Autodesk Inventor part; units mm, degrees
ref_plane "YZ Plane" through (0, 0, 0) normal (1, 0, 0) x (0, 1, 0)
ref_plane "XZ Plane" through (0, 0, 0) normal (0, 1, 0) x (-1, 0, 0)
ref_plane "XY Plane" through (0, 0, 0) normal (0, 0, 1) x (1, 0, 0)
sketch "Sketch1" plane through (0, 0, 0) normal (0, 1, 0) x (-1, 0, 0)
  line L0 (42.5, -32.5) -> (-42.5, -32.5)
  line L1 (-42.5, -32.5) -> (-42.5, 32.5)
  line L2 (-42.5, 32.5) -> (42.5, 32.5)
  line L3 (42.5, 32.5) -> (42.5, -32.5)
  point P0 (0, 0)
  point P1 (42.5, 0)
  point P2 (0, -32.5)
  dimension "d0" = 85
  dimension "d1" = 65
extrude "Extrusion1" add sketch "Sketch1" along normal blind 40
sketch "Sketch2" plane through (0, 40, 0) normal (0, 1, 0) x (1, 0, 0)
  point P0 (0, 0)
shell "Shell1" thickness 1 removed faces 1 at (14.1667, 40, 10.8333)
sketch "Sketch4" plane through (-42.5, 0, 32.5) normal (0, 0, 1) x (1, 0, 0)
  line L0 (6, 7) -> (16, 7)
  line L1 (16, 7) -> (16, 3.5)
  line L2 (16, 3.5) -> (6, 3.5)
  line L3 (6, 3.5) -> (6, 7)
  line L4 (0, 0) -> (0, 40)
  line L5 (0, 0) -> (85, 0)
  point P0 (42.5, 0)
  dimension "d7" = 10
  dimension "d8" = 3.5
  dimension "d9" = 6
  dimension "d10" = 3.5
extrude "Extrusion3" cut sketch "Sketch4" against normal blind 3
sketch "Sketch5" plane through (-42.5, 0, 32.5) normal (0, 0, 1) x (1, 0, 0)
  point P0 (42.5, 0)
fillet "Fillet1" radius 0.5 4 edges at (-26.5, 7, 32) (-36.5, 7, 32) (-26.5, 3.5, 32) (-36.5, 3.5, 32)
properties part number "timer and thermometer"
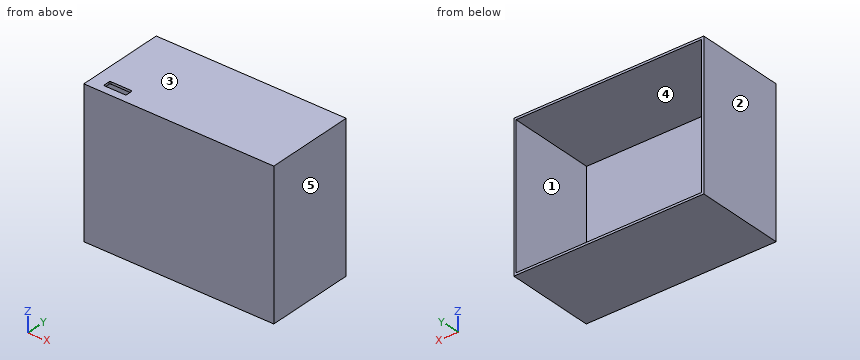
Part model, mm, in its own coordinate system. Face numbers are marked on the shaded views. A direction names the side the tool comes from. Round coordinates to 2 decimals unless told otherwise and drop trailing zeros. Order: outer loops, then holes, each group sorted by start corner. A loop starts at its lowest first (then second) coordinate and runs counter-clockwise, first axis right, second up. Notation, with made-up numbers: (-18.75, -13) -> (21.25, -13) arc R24 cw to (21.25, 18) -> close; hole circle Ø9 at (87, 7). An arc over 180 degrees is marked (long way). Put each result on its own line as item: value.
Q1. Band-saw the part on A-A (x = -28.5). Give the cut face in (y, z), and give its area (4 significant figures).
From the geometry:
outline: (0, -32.5) -> (40, -32.5) -> (40, -31.5) -> (1, -31.5) -> (1, 31.5) -> (3.5, 31.5) -> (3.5, 32.5) -> (0, 32.5) -> close; (7, 31.5) -> (40, 31.5) -> (40, 32.5) -> (7, 32.5) -> close
area: 139.5 mm2
Q2. Wall check: line 1 (X direction, y = 20.5, z = 3.5); line 2 (Z direction, x = -14, y = 34); line 3 (Y direction, x = 35.5, z = -18). Give the ranges that are in metal, low to high. Write a range as [from, to].
From the geometry:
line 1: x = [-42.5, -41.5], [41.5, 42.5]
line 2: z = [-32.5, -31.5], [31.5, 32.5]
line 3: y = [0, 1]
Q3. Band-saw the part on B-B (z = 6). Give the cut face in (x, y).
From the geometry:
outline: (-42.5, 0) -> (42.5, 0) -> (42.5, 40) -> (41.5, 40) -> (41.5, 1) -> (-41.5, 1) -> (-41.5, 40) -> (-42.5, 40) -> close
Q4. Pin check, flat tip, straight feed: pin 1 Ø19 at (x, z) = (2.5, 6.5) entering from +Y. Stop position of the tip, or through.
From the geometry:
pin 1: stops at y = 1
Q5. Band-saw the part on D-D (x = 33.5). Give the cut face in (y, z).
From the geometry:
outline: (0, -32.5) -> (40, -32.5) -> (40, -31.5) -> (1, -31.5) -> (1, 31.5) -> (40, 31.5) -> (40, 32.5) -> (0, 32.5) -> close
Q6. Band-saw the part on C-C (y = 22). Give the cut face in (x, z).
From the geometry:
outline: (-42.5, -32.5) -> (42.5, -32.5) -> (42.5, 32.5) -> (-42.5, 32.5) -> close; hole (-41.5, -31.5) -> (41.5, -31.5) -> (41.5, 31.5) -> (-41.5, 31.5) -> close
Q7. Pull direction X, two halves, no side cores. Call the marked faces 1, 2 and 3: pulls with the +X half, pulls with the -X half, needs draft (parallel to the pull), parting line crosses it, or undercut.
From the geometry:
face 1: undercut
face 2: pulls with the -X half
face 3: needs draft
Q8. Tool access for the marked faces 4 and 5: list every direction of +Z, -Z, +X, -X, +Y, -Y with a clear straight run to the whole face (end or side of a thin tool).
From the geometry:
face 4: +Y
face 5: +Z, -Z, +X, +Y, -Y
